Design review of the part built by this model. Coordinates are the model's own, in mm. A direction names the side the tool comes from. Give positions to 0.01 mm unless a question says otherwise; leave off trailing zeros. Order: outer loops, then holes, each group sorted by start corner. A loop starts at its lowest first (then second) coordinate and runs counter-clockwise, first axis right, second up. Notation, with made-up numbers: (10, -11) -> (29, -11) arc R21 ccw to (29, 13) -> close; hole circle Ø10 at (57.25, 67). An arc over 180 degrees is marked (long way). One line per item, written item: value. Start each with the question number.
1) The part is to be moulded in two halves that separate along X. For faces 1 (the face through (0.021, -5.818, 1.226)), 2 (the face through (-4.542, 6.806, 2.958)), 3 (the face through (0, 9.741, 3)), 4 (the face through (7.5, 10.8, 1.6)), say which applies: released by +X, released by -X, zero draft, split by the parting line, or undercut.
2) For pin 1 (6 mm diameter, centred on x = 5, y = -5.5, fed in from -Z); pin 2 (1.5 mm diameter, centred on y = -5.5, z = 1.5, fed in from -X); pin 3 (1.8 mm diameter, centred on y = -4.5, z = 2.5, fed in from +X); pin 4 (4 mm diameter, centred on x = -4.5, y = 6.5, fed in from -Z), all flat-tipped, find the tip position at first contact; note any pin that passes through.
3) Consider section A-A (z = 3). State the section outline as (x, y) points, plus the area to 3 significant figures.
4) Consider section C-C (x = -1). State the section outline as (y, z) points.
5) Wall thickness on line 1 along X through (y, z) = (13.75, 0.7); line 2 along X through (y, z) = (0.75, 2.4); line 3 along Y through (x, z) = (4.75, 4.5): over which ranges is each line inside the solid? List them lowest first. Write a range as from..to.
6) Consider section B-B (y = 14.25). State the section outline as (x, z) points, plus the area to 3 significant figures.
7) Tool access review of faces 5 (the face through (-1.5, -2, 3)), 6 (the face through (-2.5, 10.7, 2.3)), 7 (the face through (1.5, -2, 3)): name each direction out of +Z, -Z, +X, -X, +Y, -Y from which nothing blocks a thin tool from reaching the whole face with its end or side.
8) Consider section D-D (y = 11.5). State the section outline as (x, z) points, plus the area to 3 significant figures.
from build123d import *

# Parameters (mm, degrees)
BOSS_EXTRU_1_DEPTH      = 6
ENL_V_MAT_EXTRU_1_REACH = 24.556
ESQUISSE2_R             = 2
ESQUISSE3_R             = 2
ENL_V_MAT_EXTRU_2_DEPTH = 3


with BuildPart() as part:
    # Esquisse1 → Boss.-Extru.1 (new body)
    with BuildSketch(Plane.XY):
        Polygon((-7.5, 7.741189715), (-1.5, 5.844713829), (-1.5, -9.741189715), (1.5, -9.741189715), (1.5, 5.844713829), (7.5, 7.741189715), (7.5, 15.741189715), (2.5, 15.741189715), (2.5, 9.741189715), (-2.5, 9.741189715), (-2.5, 15.741189715), (-7.5, 15.741189715), align=None)
    extrude(amount=BOSS_EXTRU_1_DEPTH)

    # Enlèv. mat.-Extru.1: up to this face of the body (flat: up to its plane)
    enl_v_mat_extru_1_end = Plane(part.part.faces().sort_by_distance((-7.5, 11.741189715, 3))[0])
    # Esquisse2 → Enlèv. mat.-Extru.1 (cut, up to the picked face)
    with BuildSketch(Plane(origin=(7.5, 0, 0), x_dir=(0, 0, -1), z_dir=(1, 0, 0)), mode=Mode.PRIVATE) as enl_v_mat_extru_1_sk1:
        with Locations((-3, 12.741189715)):
            Circle(ESQUISSE2_R)
    enl_v_mat_extru_1_tool1 = split(extrude(enl_v_mat_extru_1_sk1.sketch, amount=-ENL_V_MAT_EXTRU_1_REACH, mode=Mode.PRIVATE), bisect_by=enl_v_mat_extru_1_end, keep=Keep.BOTH, mode=Mode.PRIVATE)
    add(enl_v_mat_extru_1_tool1.solids().sort_by(Axis((7.5, 12.74119, 3), (-1, 0, 0)))[0], mode=Mode.SUBTRACT)

    # Esquisse3 → Enlèv. mat.-Extru.2 (cut)
    with BuildSketch(Plane(origin=(1.5, 0, 0), x_dir=(0, 0, -1), z_dir=(1, 0, 0))):
        with Locations(Location((-3, -6.741189715, 0), (0, 0, 90))):
            Circle(ESQUISSE3_R)
    extrude(amount=-ENL_V_MAT_EXTRU_2_DEPTH, mode=Mode.SUBTRACT)


solid = part.part
Checked values:
1. face 1: zero draft
1. face 2: released by -X
1. face 3: undercut
1. face 4: released by +X
2. pin 1: passes through
2. pin 2: stops at x = -1.5
2. pin 3: stops at x = 1.5
2. pin 4: stops at z = 0
3. outline: (-7.5, 7.74) -> (-1.5, 5.84) -> (-1.5, -4.74) -> (1.5, -4.74) -> (1.5, 5.84) -> (7.5, 7.74) -> (7.5, 10.74) -> (2.5, 10.74) -> (2.5, 9.74) -> (-2.5, 9.74) -> (-2.5, 10.74) -> (-7.5, 10.74) -> close; (-7.5, 14.74) -> (-2.5, 14.74) -> (-2.5, 15.74) -> (-7.5, 15.74) -> close; (-1.5, -9.74) -> (1.5, -9.74) -> (1.5, -8.74) -> (-1.5, -8.74) -> close; (2.5, 14.74) -> (7.5, 14.74) -> (7.5, 15.74) -> (2.5, 15.74) -> close
3. area: 102 mm^2
4. outline: (-9.74, 0) -> (9.74, 0) -> (9.74, 6) -> (-9.74, 6) -> close; hole circle Ø4 at (-6.74, 3)
5. line 1: x = -7.5..-2.5, 2.5..7.5
5. line 2: x = -1.5..1.5
5. line 3: y = 6.87..11.42, 14.06..15.74
6. outline: (-7.5, 0) -> (-2.5, 0) -> (-2.5, 1.69) -> (-7.5, 1.69) -> close; (-7.5, 4.31) -> (-2.5, 4.31) -> (-2.5, 6) -> (-7.5, 6) -> close; (2.5, 0) -> (7.5, 0) -> (7.5, 1.69) -> (2.5, 1.69) -> close; (2.5, 4.31) -> (7.5, 4.31) -> (7.5, 6) -> (2.5, 6) -> close
6. area: 33.7 mm^2
7. face 5: +Z, -Z, -X, -Y
7. face 6: +Z, -Z, +Y
7. face 7: +Z, -Z, +X, -Y
8. outline: (-7.5, 0) -> (-2.5, 0) -> (-2.5, 1.43) -> (-7.5, 1.43) -> close; (-7.5, 4.57) -> (-2.5, 4.57) -> (-2.5, 6) -> (-7.5, 6) -> close; (2.5, 0) -> (7.5, 0) -> (7.5, 1.43) -> (2.5, 1.43) -> close; (2.5, 4.57) -> (7.5, 4.57) -> (7.5, 6) -> (2.5, 6) -> close
8. area: 28.6 mm^2
